Source: CAD feature listing. Evaluate the final solid. Frame: model axes, mm. A direction names the side the tool comes from. Coordinates: 2 decimals unless noted, no trailing zeros. Loops run counter-clockwise (first coordinate to the right, second up) from the corner with the lowest first, then second, coordinate; pieces in that order, holes last.
Item 1: Reachability of faces 4 (the flat face through (-48.342, 1, 32)), 5 (the flat face through (-28, 13, 44)), 6 (the flat face through (38, -0.371, 8)), 7 (the flat face through (-13, -8.389, 27)), 8 (the flat face through (-1, 2, 0)) from +Z, -Z, +X, -X, +Y, -Y: full face, straight path, thin tool, end or side. Return the list, or none.
Item 2: Section query A-A, the plane y = 24. Return the cut outline in (x, z), then the cut area to 3 significant figures.
Item 3: Section query D-D, the plane y = 13.5. Return the cut outline in (x, z), then the cut area to 3 significant figures.
Item 4: Line query: probe 1 along Y at (x, z) = (-37, 18); probe 2 along Y at (x, z) = (12, 25); probe 3 along Z at (x, y) = (14, 18.5). Output: solid intervals per line, ascending.
Item 5: Pull-direction query (Y, two-part tool) for faces 1 (the flat face through (-12, -30.409, 12)), 2 (the cylindrical face through (19.66, -8.2, 8.11)), 3 (the flat face through (-40, 18, 64)); classes: +Y half, -Y half, draft (parallel to the pull), parting line (faces both ways), or undercut.
Item 6: Pin query (flat end, axial travel): pin 1 Ø6.5 at (x, y) = (5, 16) entering from +Z; pin 2 Ø12 at (x, y) = (-17, -4) entering from +Z; pin 3 Ø14 at (y, z) = (1, 27) entering from +X. Return the tip coordinate at first contact, or that it passes through.
Item 7: Section query B-B, the plane z = 7. Return the cut outline in (x, y), then the cut area to 3 significant figures.
```python
from build123d import *

# Parameters (mm, degrees)
F0_W      = 96
F0_H      = 64
F1_DEPTH  = 16
F2_W      = 16
F2_H      = 64
F3_DEPTH  = 48
F4_R      = 32
F5_W      = 40
F5_H      = 42
F6_DEPTH  = 28
F7_W      = 40
F7_H      = 12
F8_DEPTH  = 28
F10_DEPTH = 25.4
F11_R     = 12
F12_DEPTH = 63.246
F14_DEPTH = 25.4


with BuildPart() as f1:
    # F0 (on Top) → F1 (new body)
    with BuildSketch(Plane.XY):
        with Locations((-0.3420451991, 1.5907883644)):
            Rectangle(F0_W, F0_H)
    extrude(amount=F1_DEPTH)

    # F2 (on face) → F3 (join)
    with BuildSketch(Plane.XY.offset(16)):
        with Locations((-40.3420451991, 1.5907883644)):
            Rectangle(F2_W, F2_H)
    extrude(amount=F3_DEPTH)

    # F4
    f4_edges = [f1.edges().sort_by_distance(p)[0] for p in [
        (-40.342045, -30.409212, 64),
    ]]
    fillet(f4_edges, radius=F4_R)

    # F5 (on face) → F6 (join)
    with BuildSketch(Plane.XY.offset(16)):
        with Locations((-12.3420451991, 12.61113044)):
            Rectangle(F5_W, F5_H)
    extrude(amount=F6_DEPTH)

    # F7 (on face) → F8 (join)
    with BuildSketch(Plane.XY.offset(16)):
        with Locations((27.6579548009, 27.5907883644)):
            Rectangle(F7_W, F7_H)
    extrude(amount=F8_DEPTH)

    # F9 (on face) → F10 (cut)
    with BuildSketch(Plane.XZ.offset(-21.5907883644)):
        Polygon((47.6579548009, 44), (7.6579548009, 44), (47.6579548009, 16), align=None)
    extrude(amount=-F10_DEPTH, mode=Mode.SUBTRACT)

    # F11 (on face) → F12 (cut)
    with BuildSketch(Plane.XZ.offset(8.38886956)):
        with Locations((-12.3420451991, 44)):
            Circle(F11_R)
    extrude(amount=-F12_DEPTH, mode=Mode.SUBTRACT)

    # F13 (on face) → F14 (cut)
    with BuildSketch(Plane.XY.offset(16)):
        with BuildLine():
            ThreePointArc((35.6579548009, -8.3714298824), (33.3148090504, -2.714575633), (27.6579548009, -0.3714298824))
            Line((27.6579548009, -0.3714298824), (27.6579548009, -16.3714298824))
            ThreePointArc((27.6579548009, -16.3714298824), (33.3148090504, -14.0282841319), (35.6579548009, -8.3714298824))
        make_face()
        with BuildLine():
            Line((47.6579548009, -0.3714298824), (27.6579548009, -0.3714298824))
            ThreePointArc((27.6579548009, -0.3714298824), (33.3148090504, -2.714575633), (35.6579548009, -8.3714298824))
            ThreePointArc((35.6579548009, -8.3714298824), (33.3148090504, -14.0282841319), (27.6579548009, -16.3714298824))
            Line((27.6579548009, -16.3714298824), (47.6579548009, -16.3714298824))
            Line((47.6579548009, -16.3714298824), (47.6579548009, -0.3714298824))
        make_face()
        with BuildLine():
            Line((27.6579548009, -16.3714298824), (27.6579548009, -0.3714298824))
            ThreePointArc((27.6579548009, -0.3714298824), (19.6579548009, -8.3714298824), (27.6579548009, -16.3714298824))
        make_face()
    extrude(amount=-F14_DEPTH, mode=Mode.SUBTRACT)


solid = f1.part
```
Verdict:
1. face 4: +Z, -Z, -X, +Y, -Y
1. face 5: +Z, +X, +Y, -Y
1. face 6: +Z, -Z, +X
1. face 7: +Z, +X, -Y
1. face 8: -Z, +X, -X, +Y, -Y
2. outline: (-48.34, 0) - (47.66, 0) - (47.66, 16) - (7.66, 44) - (-0.34, 44) arc R12 cw to (-24.34, 44) - (-32.34, 44) - (-32.34, 64) - (-48.34, 64) - close
2. area: 3,760 mm2
3. outline: (-48.34, 0) - (47.66, 0) - (47.66, 16) - (7.66, 16) - (7.66, 44) - (-0.34, 44) arc R12 cw to (-24.34, 44) - (-32.34, 44) - (-32.34, 64) - (-48.34, 64) - close
3. area: 3,200 mm2
4. probe 1: y = -30.41 to 33.59
4. probe 2: y = 21.59 to 33.59
4. probe 3: z = 0 to 16
5. face 1: -Y half
5. face 2: undercut
5. face 3: draft
6. pin 1: stops at z = 44
6. pin 2: stops at z = 38.49
6. pin 3: stops at x = 7.66
7. outline: (-48.34, -30.41) - (47.66, -30.41) - (47.66, -16.37) - (27.66, -16.37) arc R8 cw to (27.66, -0.37) - (47.66, -0.37) - (47.66, 33.59) - (-48.34, 33.59) - close
7. area: 5,720 mm2
